```python
from build123d import *

# Parameters (mm, degrees)
BODY_DEPTH   = 33.32
POCKET_DEPTH = 24.32
SKETCH3_R    = 4.2
HOLESX_DEPTH = 6.35
SKETCH4_R    = 4.2
HOLESY_DEPTH = 6.35


with BuildPart() as part:
    # Sketch1 → Body (new body)
    with BuildSketch(Plane.XY.offset(-16.66)):
        Polygon((0, 0), (38.1, 0), (38.1, 6.35), (6.35, 38.1), (0, 38.1), align=None)
    extrude(amount=BODY_DEPTH)

    # Sketch2 → Pocket (cut)
    with BuildSketch(Plane.XY.offset(12.16)):
        Polygon((6.35, 6.35), (48.1, 6.35), (6.35, 48.1), align=None)
    extrude(amount=-POCKET_DEPTH, mode=Mode.SUBTRACT)

    # Sketch3 → HolesX (cut)
    with BuildSketch(Plane(origin=(0, 6.35, 0), x_dir=(1, 0, 0), z_dir=(0, 1, 0))):
        with Locations(Location((19.05, 0, 0), (0, 0, 270))):
            Circle(SKETCH3_R)
    extrude(amount=-HOLESX_DEPTH, mode=Mode.SUBTRACT)

    # Sketch4 → HolesY (cut)
    with BuildSketch(Plane(origin=(6.35, 0, 0), x_dir=(0, 0, -1), z_dir=(1, 0, 0))):
        with Locations((0, 19.05)):
            Circle(SKETCH4_R)
    extrude(amount=-HOLESY_DEPTH, mode=Mode.SUBTRACT)


solid = part.part
```
Verification items for the finished model (mm, model axes). A direction names the side the tool comes from. Give positions to 0.01 mm unless a question says otherwise; leave off trailing zeros. Order: outer loops, then holes, each group sorted by start corner. A loop starts at its lowest first (then second) coordinate and runs counter-clockwise, first axis right, second up. Notation, with made-up numbers: M 35.5,68 L 83.5,68 A13 cw 83.5,80 Z; hole C -34.5,-25.5 d9. An arc over 180 degrees is marked long. Return JSON: item names as keys, results as strings. Group by question number.
1) Section check A-A on y = 19.05. Record the cut outline in (x, z), and give its area (3 significant figures).
2) Section check D-D on y = 24. Record the cut outline in (x, z), and give its area (3 significant figures).
3) Scan lines: line 1 (X direction, y = 1, z = 0); line 2 (Z direction, x = 13, y = 18). Record each from-to range of solid material in increasing order.
4) Go/stop test with flat-tipped pins: pin 1 Ø7.5 at (x, z) = (18, -3) entering from +Y; pin 2 Ø6.5 at (x, z) = (19.05, 0) entering from -Y; pin 3 Ø3 at (y, z) = (10.5, 10) entering from +X. Record where each tip stops, or that it passes through.
5) Mould release check, pull along Z, two halves, no side actions. Record for faces 3 (the face through (3.22, 14.95, 0.91)), 4 (the face through (3, 38.1, 0)), 5 (the face through (15, 15, 12.16)), 6 (the face through (15, 15, -16.66)): pulls with the +Z half, pulls with the -Z half, needs draft (parallel to the pull), parting line crosses it, or undercut.
6) Access from +Z, -Z, +X, -X, +Y, -Y to the whole of each face (thin tool, end or side, straight path). Record for faces 1 (the face through (26, 6.35, 0)), 2 (the face through (0, 24, 0)).
7) Section check B-B on z = 0. Record the cut outline in (x, y), and give its area (3 significant figures).
Answer block:
{
 "1": {"outline": "M 0,-16.66 L 25.4,-16.66 L 25.4,-12.16 L 6.35,-12.16 L 6.35,-4.2 L 0,-4.2 Z; M 0,4.2 L 6.35,4.2 L 6.35,12.16 L 25.4,12.16 L 25.4,16.66 L 0,16.66 Z", "area": "330 mm^2"},
 "2": {"outline": "M 0,-16.66 L 20.45,-16.66 L 20.45,-12.16 L 6.35,-12.16 L 6.35,12.16 L 20.45,12.16 L 20.45,16.66 L 0,16.66 Z", "area": "338 mm^2"},
 "3": {"line 1": "x = 0 to 14.85, 23.25 to 38.1", "line 2": "z = -16.66 to -12.16, 12.16 to 16.66"},
 "4": {"pin 1": "stops at y = 6.35", "pin 2": "passes through", "pin 3": "stops at x = 6.35"},
 "5": {"face 3": "undercut", "face 4": "needs draft", "face 5": "undercut", "face 6": "pulls with the -Z half"},
 "6": {"face 1": "+X, +Y", "face 2": "+Z, -Z, -X, +Y, -Y"},
 "7": {"outline": "M 0,0 L 14.85,0 L 14.85,6.35 L 6.35,6.35 L 6.35,14.85 L 0,14.85 Z; M 0,23.25 L 6.35,23.25 L 6.35,38.1 L 0,38.1 Z; M 23.25,0 L 38.1,0 L 38.1,6.35 L 23.25,6.35 Z", "area": "337 mm^2"}
}
